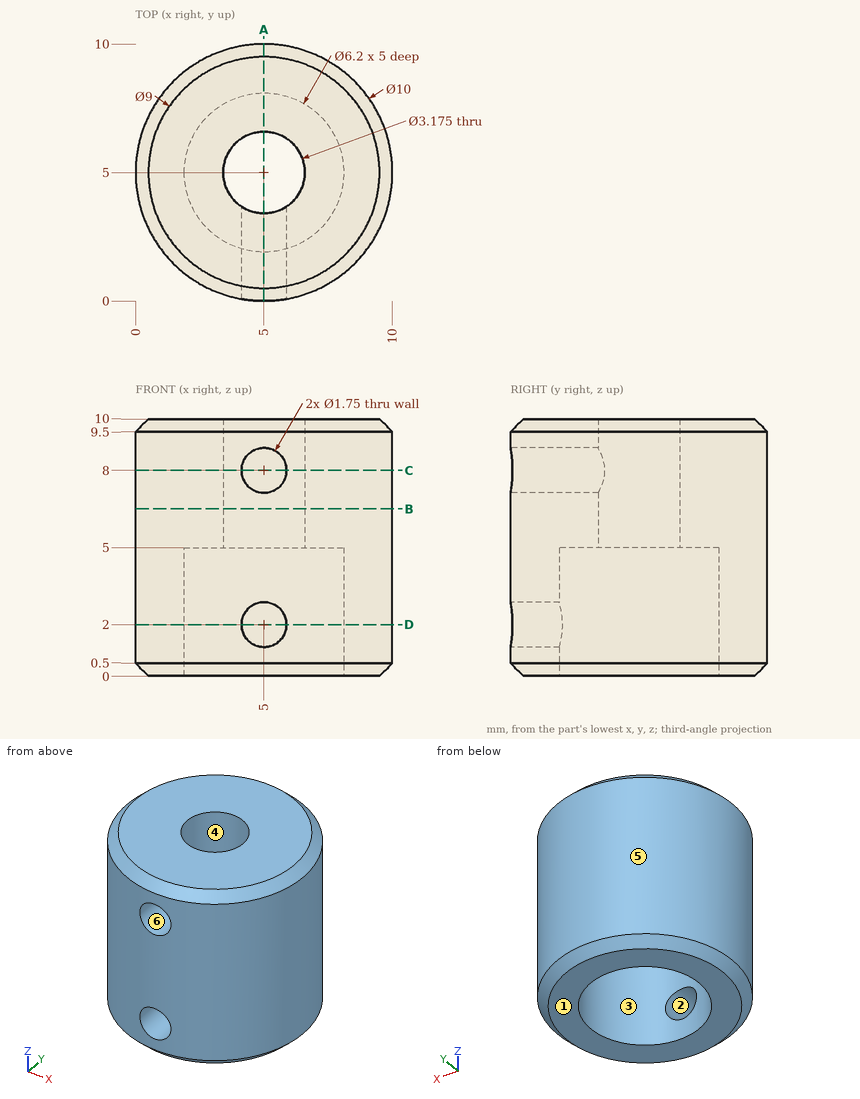
Verification items for this drawing (mm, ordinates from the low corner). A direction names the side the tool comes from. Coordinates: 2 decimals unless noted, no trailing zeros. Write each loop counter-clockwise with the first axis right and the second up, starting at its lowest first coordinate (ties: lowest second). Pieces come first, ordered by that corner, then holes. Notation, with made-up numbers: M 24.5,46.25 L 82.5,46.25 A16 cw 82.5,52.25 Z; hole C 75,-36 d11. An arc over 180 degrees is marked long. One line per item, written item: value. Start each with the question number.
(1) Sectioned sample at C-C, the plane z = 8. Enter the section's corners in (x, y) (1 decimal), and give its area (3 significant figures).
(2) Depth check by flat-ended pin: pin 1 (1.5 mm diameter, centred on x = 3.5, z = 3, fed in from -Y); pin 2 (3 mm diameter, centred on x = 5, y = 4, fed in from -Z); pin 3 (1.6 mm diameter, centred on x = 5, z = 8, fed in from -Y). Enter the tip coordinate at first touch or a pass-through.
(3) Sectioned sample at B-B, the plane z = 6.5. Enter the section's corners in (x, y) (1 decimal), and give its area (3 significant figures).
(4) Sectioned sample at D-D, the plane z = 2. Enter the section's corners in (x, y) (3 decimals), and give its area (3 significant figures).
(5) Sectioned sample at A-A, the plane x = 5. Enter the section's corners in (y, z) (1 decimal), and give its area (3 significant figures).
(6) Release check for a two-part mould opening along Y. For the marked faces 4, 5 and 6 record: released by +Y, released by -Y, zero draft, split by the parting line, or undercut.
(7) Scan lines: line 1 along Z through (x, y) = (5, 1.4) (3 decimals); line 2 along Y through (x, z) = (5, 3.9); line 3 along Y through (x, z) = (5, 6.8). Record each from-to range of solid material in increasing order. Write a range as [from, to].
(8) Tool access check on the marked faces 1, 2 and 3. Record the directions out of +Z, -Z, +X, -X, +Y, -Y that give a thin tool (end or side, any length) a straight path to the whole face; none if there is none.
Filled sheet:
1. outline: M 4.1,0.1 L 4.1,3.7 A1.6 cw long 5.9,3.7 L 5.9,0.1 A5 ccw long Z
1. area: 64.5 mm²
2. pin 1: y = 0.06
2. pin 2: z = 5
2. pin 3: y = 6.37
3. outline: C 5,5 d10; hole C 5,5 d3.2
3. area: 70.6 mm²
4. outline: M 4.125,0.077 L 4.125,2.026 A3.1 cw long 5.875,2.026 L 5.875,0.077 A5 ccw long Z
4. area: 45.0 mm²
5. outline: M 0,0.5 L 0.5,0 L 1.9,0 L 1.9,1.1 L 0,1.1 Z; M 0,2.9 L 1.9,2.9 L 1.9,5 L 3.4,5 L 3.4,7.1 L 0,7.1 Z; M 0,8.9 L 3.4,8.9 L 3.4,10 L 0.5,10 L 0,9.5 Z; M 6.6,5 L 8.1,5 L 8.1,0 L 9.5,0 L 10,0.5 L 10,9.5 L 9.5,10 L 6.6,10 Z
5. area: 43.3 mm²
6. face 4: undercut
6. face 5: split by the parting line
6. face 6: zero draft
7. line 1: [0, 1.125], [2.875, 7.125], [8.875, 10]
7. line 2: [0, 1.9], [8.1, 10]
7. line 3: [0, 3.41], [6.59, 10]
8. face 1: -Z, +X, -X, +Y, -Y
8. face 2: -Y
8. face 3: -Z
